Check sheet for the modelled part. Datum: model origin and axes. Units: mm. A direction names the side the tool comes from. Give positions to 0.01 mm unless a question says otherwise; leave off trailing zeros. Loops run counter-clockwise (first coordinate to the right, second up) from the corner with the lowest first, then second, coordinate; pieces in that order, holes last. Notation, with made-up numbers: (-21, -16) -> (18, -16) arc R34 ccw to (18, 16) -> close; hole circle Ø10 at (24, 88). An arc over 180 degrees is marked (long way). Answer as CSV lines item,"result". Start each with the question number.
(1) Section check C-C on x = 20.5. Enter the section's corners in (y, z) (3 decimals), plus the area to 3 significant figures.
(2) Section check D-D on z = -33.5. Enter the section's corners in (x, y) (3 decimals).
(3) Section check A-A on z = -55. Enter the section's corners in (x, y) (3 decimals), plus the area to 3 significant figures.
(4) Access from +Z, -Z, +X, -X, +Y, -Y to the whole of each face (thin tool, end or side, straight path). Record for faces 1 (the face through (16, 5.25, -56)), 2 (the face through (32.65, 3, -30)), 3 (the face through (16, 2, -35)).
(5) Material ranges on line 1 (Z direction, x = 20, y = 5); line 2 (X direction, y = 1, z = -7); line 3 (Z direction, x = 12, y = 0.5), recorded low to high. Write a range as from..to.
(6) Release check for a two-part mould opening along X. For faces 4 (the face through (16, 6.25, -30)), 5 (the face through (20.398, 2.077, -56.32)), 6 (the face through (11.175, 3, -56)), 7 (the face through (0, 3, -30)) record: pulls with the +X half, pulls with the -X half, needs draft (parallel to the pull), parting line crosses it, or undercut.
(7) Gauge pin test, flat end, axial feed: pin 1 Ø2 at (x, y) = (20, 2) entering from +Z. Record the tip position at first contact, or that the pin passes through.
(8) Section check B-B on y = 1.75. Enter the section's corners in (x, z) (3 decimals), plus the area to 3 significant figures.
from build123d import *

# Parameters (mm, degrees)
SKETCH1_W               = 61.25
SKETCH1_H               = 6.25
BOSS_EXTRUDE1_DEPTH     = 32.65
CUT_EXTRUDE1_DEPTH      = 70.689651312
CUT_EXTRUDE1_DEPTH_BACK = 35
CUT_EXTRUDE2_DEPTH      = 10
FILLET1_R               = 3


with BuildPart() as part:
    # Sketch1 → Boss-Extrude1 (new body)
    with BuildSketch(Plane(origin=(0, 0, 0), x_dir=(0, 0, -1), z_dir=(1, 0, 0))):
        with Locations((30.625, 3.125)):
            Rectangle(SKETCH1_W, SKETCH1_H)
    extrude(amount=BOSS_EXTRUDE1_DEPTH)

    # Sketch2 → Cut-Extrude1 (cut, two sides: drawn at the far end of the back side and taken through both)
    with BuildSketch(Plane.XY.offset(-CUT_EXTRUDE1_DEPTH_BACK)):
        with BuildLine():
            Line((5, 0), (27.65, 0))
            ThreePointArc((27.65, 0), (16.325, 4.25), (5, 0))
        make_face()
    extrude(amount=CUT_EXTRUDE1_DEPTH + CUT_EXTRUDE1_DEPTH_BACK, mode=Mode.SUBTRACT)

    # Sketch3 → Cut-Extrude2 (cut)
    with BuildSketch(Plane(origin=(0, 0, -61.25), x_dir=(-1, 0, 0), z_dir=(0, 0, -1))):
        Polygon((-11.175, 1), (-11.175, 5.25), (-21.475, 5.25), (-19.35, 3.125), (-21.475, 1), align=None)
    extrude(amount=-CUT_EXTRUDE2_DEPTH, mode=Mode.SUBTRACT)

    # Fillet1
    fillet1_edges = [part.edges().sort_by_distance(p)[0] for p in [
        (32.65, 3.125, 0),
        (0, 3.125, 0),
        (0, 3.125, -61.25),
        (32.65, 3.125, -61.25),
    ]]
    fillet(fillet1_edges, radius=FILLET1_R)


solid = part.part
Working result:
1,outline,"(0, -61.25) -> (1, -61.25) -> (1, -51.25) -> (1.975, -51.25) -> (1.975, -61.25) -> (4.275, -61.25) -> (4.275, -51.25) -> (5.25, -51.25) -> (5.25, -61.25) -> (6.25, -61.25) -> (6.25, 0) -> (3.736, 0) -> (3.736, -35) -> (0, -35) -> close"
1,area,"233 mm^2"
2,outline,"(0, 0) -> (5, 0) arc R17.214 cw to (27.65, 0) -> (32.65, 0) -> (32.65, 6.25) -> (0, 6.25) -> close"
3,outline,"(0, 0) -> (32.65, 0) -> (32.65, 6.25) -> (0, 6.25) -> close; hole (11.175, 1) -> (21.475, 1) -> (19.35, 3.125) -> (21.475, 5.25) -> (11.175, 5.25) -> close"
3,area,"165 mm^2"
4,face 1,"-Z"
4,face 2,"+Z, -Z, +X, +Y, -Y"
4,face 3,"+Z, -Y"
5,line 1,"z = -51.25..0"
5,line 2,"x = 0..6.26, 26.39..32.65"
5,line 3,"z = -61.25..-35"
6,face 4,"needs draft"
6,face 5,"undercut"
6,face 6,"undercut"
6,face 7,"pulls with the -X half"
7,pin 1,"stops at z = -35"
8,outline,"(0, -58.25) arc R3 ccw to (3, -61.25) -> (11.175, -61.25) -> (11.175, -51.25) -> (20.725, -51.25) -> (20.725, -61.25) -> (29.65, -61.25) arc R3 ccw to (32.65, -58.25) -> (32.65, -3) arc R3 ccw to (29.65, 0) -> (25.259, 0) -> (25.259, -35) -> (7.391, -35) -> (7.391, 0) -> (3, 0) arc R3 ccw to (0, -3) -> close"
8,area,"1,270 mm^2"
